Geometry: final body of the model. Coordinates: model frame, mm. A direction names the side the tool comes from. Coordinates: 2 decimals unless noted, no trailing zeros. Loops run counter-clockwise (first coordinate to the right, second up) from the corner with the lowest first, then second, coordinate; pieces in that order, holes last. Notation, with made-up numbers: (80, -27.75) -> (101, -27.75) arc R14 ccw to (101, -7.75) -> close; hole circle Ø11 at (8.5, 1.25). An arc over 180 degrees is marked (long way). One line per item, written item: value. Start each with the question number.
Item 1: Section query B-B on x = 0. Return loops of the section in (y, z), then the cut area to 3 significant figures.
Item 2: Ray query, probe 1 along X at (y, z) = (-5.75, 0); probe 2 along Y at (x, z) = (-20.5, 3); probe 3 along X at (y, z) = (0, 0). Return the intervals inside material, ascending. Write a range as from..to.
Item 3: Section query D-D on y = 10. Return loops of the section in (x, z), then the cut area to 3 significant figures.
Item 4: Section query C-C on y = 0.5. Return loops of the section in (x, z).
Item 5: Section query A-A on z = 0. Return loops of the section in (x, y).
Item 6: Contact query for flat-ended pins moving along their axis: pin 1 Ø4 at (y, z) = (-10, 6.5) entering from -X; pin 2 Ø6 at (x, y) = (25.5, -0.5) entering from -Z; pin 3 Ø10 at (y, z) = (0.5, 23.5) entering from +X. Output: stop coordinate, or through.
Item 7: Set-up query: faces 4 (the flat face through (16, 3.5, 8)), 5 (the cylindrical face through (6.31, -9.42, 20.03)), 6 (the flat face through (-16, 15.5, -16)). Return all of +Z, -Z, +X, -X, +Y, -Y with unobstructed straight access to the full face (end or side cutting, diameter ignored); none if empty.
Item 8: Mould query, pull axis Z, two halves, no side actions, for faces 1 (the cylindrical face through (-10.648, 0.049, -13.887)), 2 (the flat face through (-16, -15.5, 16)), 3 (the cylindrical face through (-39.05, -0.19, -8.67)). Classes: +Z half, -Z half, draft (parallel to the pull), parting line (faces both ways), or undercut.
from build123d import *


with BuildPart() as f1:
    # F0 (on Right) → F1 (revolve)
    with BuildSketch(Plane.YZ):
        with BuildLine():
            Line((-15.5, 38), (-15.5, 21))
            Line((-15.5, 21), (-3.5, 21))
            Line((-3.5, 21), (-3.5, 17.5))
            Line((-3.5, 17.5), (3.5, 17.5))
            Line((3.5, 17.5), (3.5, 21))
            Line((3.5, 21), (15.5, 21))
            Line((15.5, 21), (15.5, 38))
            ThreePointArc((15.5, 38), (14.914214, 39.414214), (13.5, 40))
            Line((13.5, 40), (-13.5, 40))
            ThreePointArc((-13.5, 40), (-14.914214, 39.414214), (-15.5, 38))
        make_face()
    revolve(axis=Axis((0, 5.437174, 0), (0, 1, 0)))


solid = f1.part
Reply:
1. outline: (-15.5, -38) arc R2 ccw to (-13.5, -40) -> (13.5, -40) arc R2 ccw to (15.5, -38) -> (15.5, -21) -> (3.5, -21) -> (3.5, -17.5) -> (-3.5, -17.5) -> (-3.5, -21) -> (-15.5, -21) -> close; (-15.5, 21) -> (-3.5, 21) -> (-3.5, 17.5) -> (3.5, 17.5) -> (3.5, 21) -> (15.5, 21) -> (15.5, 38) arc R2 ccw to (13.5, 40) -> (-13.5, 40) arc R2 ccw to (-15.5, 38) -> close
1. area: 1,220 mm²
2. probe 1: x = -40..-21, 21..40
2. probe 2: y = -3.5..3.5
2. probe 3: x = -40..-17.5, 17.5..40
3. outline: circle Ø80 at (0, 0); hole circle Ø42 at (0, 0)
3. area: 3,640 mm²
4. outline: circle Ø80 at (0, 0); hole circle Ø35 at (0, 0)
5. outline: (-40, -13.5) arc R2 ccw to (-38, -15.5) -> (-21, -15.5) -> (-21, -3.5) -> (-17.5, -3.5) -> (-17.5, 3.5) -> (-21, 3.5) -> (-21, 15.5) -> (-38, 15.5) arc R2 ccw to (-40, 13.5) -> close; (17.5, -3.5) -> (21, -3.5) -> (21, -15.5) -> (38, -15.5) arc R2 ccw to (40, -13.5) -> (40, 13.5) arc R2 ccw to (38, 15.5) -> (21, 15.5) -> (21, 3.5) -> (17.5, 3.5) -> close
6. pin 1: stops at x = -39.75
6. pin 2: stops at z = -33.07
6. pin 3: stops at x = 35.46
7. face 4: +Y
7. face 5: -Y
7. face 6: +Z, -Z, +X, -X, +Y
8. face 1: undercut
8. face 2: draft
8. face 3: parting line
